Source: CAD feature listing. Evaluate the final solid. Frame: model axes, mm. A direction names the side the tool comes from. Give positions to 0.01 mm unless a question says otherwise; leave off trailing zeros. Order: outer loops, then holes, each group sorted by start corner. A loop starts at its lowest first (then second) coordinate and runs counter-clockwise, first axis right, second up. Notation, with made-up numbers: M -10.5,51.5 L -4.5,51.5 A23 ccw -4.5,73.5 Z; hole C 8.25,63.25 d3. An arc over 180 degrees is marked long. Use CSV: the item, a comma, the result in double quotes. Start each with the question number.
1. Section query D-D, the plane x = -6.5. Return the cut outline in (y, z), plus the area to 3 significant figures.
2. Pin query (flat end, axial travel): P1, Ø1, axis at x = 3, y = 3, coming from the +Z side; P2, Ø3, axis at y = 3.5, z = 12, coming from the +X side; P3, Ø7, axis at x = 1.5, z = 10.5, coming from the -Y side. Return the tip coordinate at first contact, or that it passes through.
3. Section query B-B, the plane z = 12.25. Return the cut outline in (x, y), plus the area to 3 significant figures.
4. Section query C-C, the plane y = 13. Return the cut outline in (x, z), plus the area to 3 significant figures.
5. Reachability of faces 1 (the flat face through (3, 1.75, 14)), 2 (the cylindrical face through (-0.07, 12.46, 10.75)), 3 (the flat face through (10, -6, 10)) from +Z, -Z, +X, -X, +Y, -Y: full face, straight path, thin tool, end or side. Return the list, or none.
6. Line query: line 1 along X through (y, z) = (4.25, 11.5); line 2 along Y through (x, z) = (1, 10.5); line 3 along Y through (x, z) = (4.75, 15.5). Output: solid intervals per line, ascending. Write a range as [from, to].
7. Section query A-A, the plane x = 0. Return the cut outline in (y, z), plus the area to 3 significant figures.
8. Mould query, pull axis Y, two halves, no side actions, for faces 4 (the flat face through (0, -2, 24.5)), 5 (the cylindrical face through (0.14, -11.04, 13.59)), 6 (the cylindrical face through (0, 1, 9)). Classes: released by +Y, released by -Y, zero draft, split by the parting line, or undercut.
from build123d import *

# Parameters (mm, degrees)
F1_DEPTH = 10
F5_R     = 2


with BuildPart() as f1:
    # F0 (on Right) → F1 (new body, symmetric)
    with BuildSketch(Plane.YZ):
        with BuildLine():
            Line((-15, 0), (0, 0))
            Line((0, 0), (0, 24.5))
            Line((0, 24.5), (-5, 24.5))
            ThreePointArc((-5, 24.5), (-11.367509, 12.808167), (-15, 0))
        make_face()
    extrude(amount=F1_DEPTH, both=True)

    # F3 (on Right) → F4 (revolve)
    with BuildSketch(Plane.YZ):
        Polygon((0, 12.25), (15, 12.25), (15, 13.75), (10, 13.75), (1.75, 16.75), (1.75, 15.5), (0, 15.5), align=None)
    revolve(axis=Axis((0, 7.5, 12.25), (0, -1, 0)))

    # F5
    f5_edges = [f1.edges().sort_by_distance(p)[0] for p in [
        (0, -5, 24.5),
        (0, -15, 0),
        (0, 0, 0),
    ]]
    fillet(f5_edges, radius=F5_R)


solid = f1.part
Result set:
1,outline,"M -14.55,2.41 A2 ccw -12.59,0 L -2,0 A2 ccw 0,2 L 0,24.5 L -3.95,24.5 A2 ccw -5.61,23.62 A60 ccw Z"
1,area,"269 mm2"
2,P1,"z = 15.49"
2,P2,"x = 4.41"
2,P3,"y = -13.4"
3,outline,"M -10,-11.59 L 10,-11.59 L 10,0 L 3.25,0 L 3.25,1.75 L 4.5,1.75 L 1.5,10 L 1.5,15 L -1.5,15 L -1.5,10 L -4.5,1.75 L -3.25,1.75 L -3.25,0 L -10,0 Z"
3,area,"308 mm2"
4,outline,"C 0,12.25 d3"
4,area,"7.07 mm2"
5,face 1,"none"
5,face 2,"+Y"
5,face 3,"+Z, -Z, +X, +Y, -Y"
6,line 1,"[-3.51, 3.51]"
6,line 2,"[-12.25, 8.58]"
6,line 3,"[-10.19, 0]"
7,outline,"M -14.55,2.41 A2 ccw -12.59,0 L -2,0 A2 ccw 0,2 L 0,9 L 1.75,9 L 1.75,7.75 L 10,10.75 L 15,10.75 L 15,13.75 L 10,13.75 L 1.75,16.75 L 1.75,15.5 L 0,15.5 L 0,24.5 L -3.95,24.5 A2 ccw -5.61,23.62 A60 ccw Z"
7,area,"345 mm2"
8,face 4,"zero draft"
8,face 5,"released by -Y"
8,face 6,"undercut"
